Drawing for the job (mm, zero at the part's lowest x, y, z). Coordinates: 2 decimals unless noted, no trailing zeros. Order: outer loops, then holes, each group sorted by start corner. A loop starts at its lowest first (then second) coordinate and runs counter-clockwise, first axis right, second up.
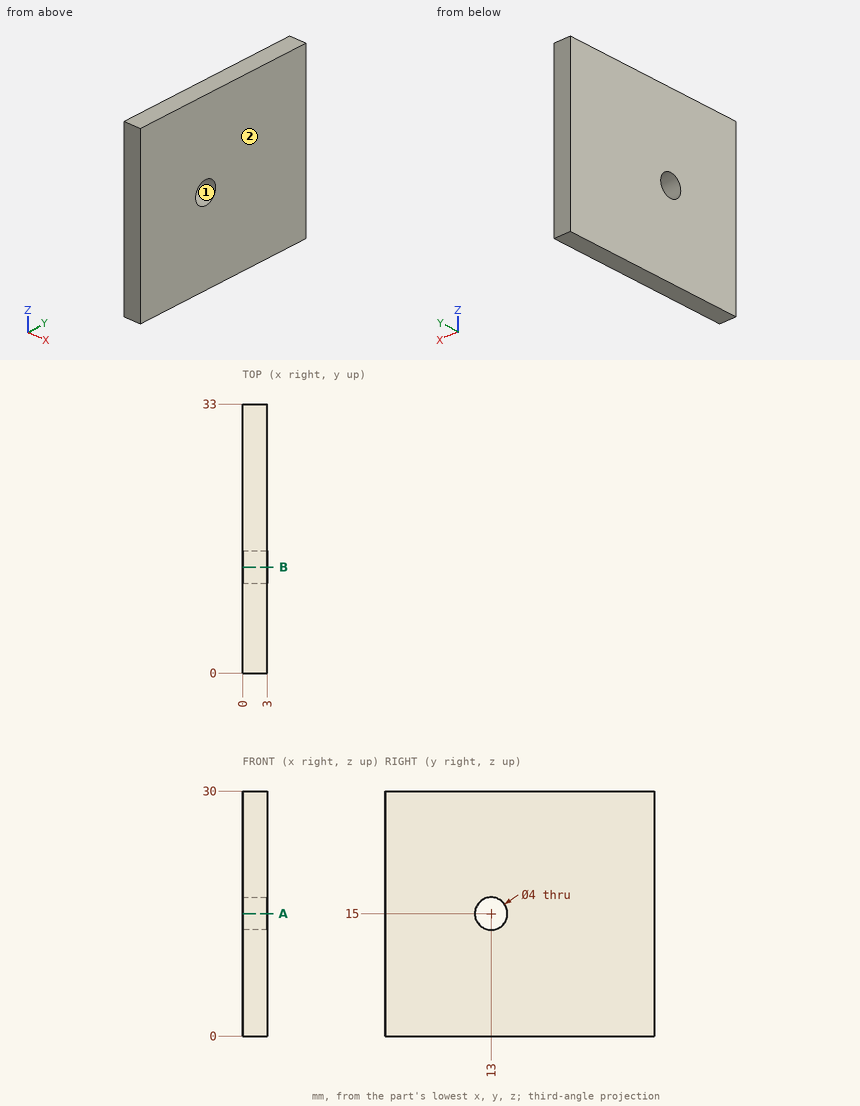
(1) Slice it at B-B, the plane y = 13. Give the cut face in (x, z).
(2) Pull direction Z, two halves, no side cores. Call the marked faces 1 and 2: +Z half, -Z half, draft (parallel to the pull), parting line (faces both ways), or undercut.
(3) Probe line 1 (Y direction, x = 1.5, z = 15); line 2 (Y direction, x = 1.1, z = 16.25); line 3 (Z direction, x = 0.5, y = 12). List the from-to ranges inside material, lowest first.
(4) Slice it at A-A, the plane z = 15. Give the cut face in (x, y).
Here are the results:
1. outline: (0, 0) - (3, 0) - (3, 13) - (0, 13) - close; (0, 17) - (3, 17) - (3, 30) - (0, 30) - close
2. face 1: undercut
2. face 2: draft
3. line 1: y = 0 to 11, 15 to 33
3. line 2: y = 0 to 11.44, 14.56 to 33
3. line 3: z = 0 to 13.27, 16.73 to 30
4. outline: (0, 0) - (3, 0) - (3, 11) - (0, 11) - close; (0, 15) - (3, 15) - (3, 33) - (0, 33) - close
